Here's the drawing with two shaded views (mm, measured from the low corner). I have some questions. A direction names the side the tool comes from. Round coordinates to 2 decimals unless told otherwise and drop trailing zeros. Loops run counter-clockwise (first coordinate to the right, second up) from the corner with the lowest first, then second, coordinate; pieces in that order, holes last.
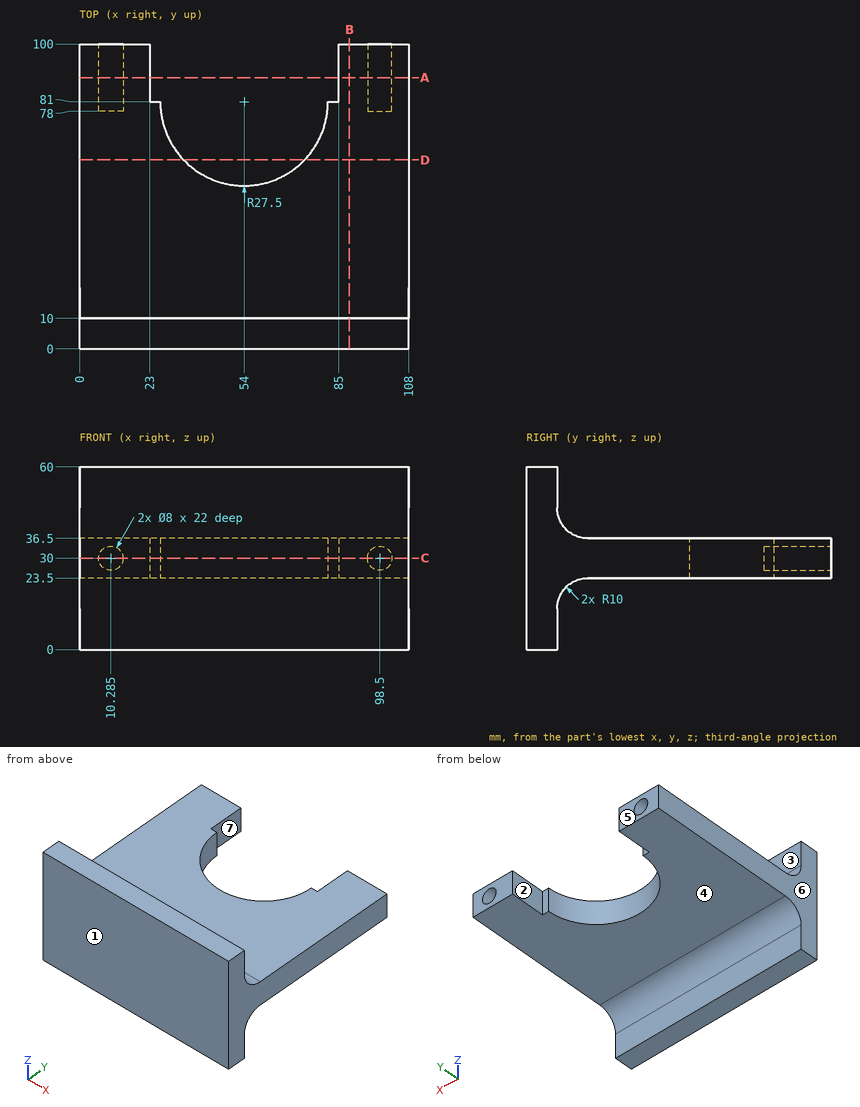
(1) If we section it at C-C, the plane z = 30: List the corners of the cut face in (x, y) for me (1 decimal).
Worked answers:
outline: (0, 0) - (108, 0) - (108, 100) - (102.5, 100) - (102.5, 78) - (94.5, 78) - (94.5, 100) - (85, 100) - (85, 81) - (81.5, 81) arc R27.5 cw to (26.5, 81) - (23, 81) - (23, 100) - (14.3, 100) - (14.3, 78) - (6.3, 78) - (6.3, 100) - (0, 100) - close
(2) If I drill on line 1 (Z direction, x = 98.5, y = 91.75); line 2 (Z direction, x = 101, y = 75.5); line 3 (Y direction, x = 68, z = 52.5), over which ranges is the centre line in solid material (lowest first)?
Worked answers:
line 1: z = 23.5 to 26, 34 to 36.5
line 2: z = 23.5 to 36.5
line 3: y = 0 to 10
(3) Will these pins go through, and if not, where does the flat tip stop? P1, Ø3, axis at x = 24, z = 27.5, coming from the +Y side; P2, Ø12, axis at x = 97, y = 18, coming from the +Z side; P3, Ø1.5, axis at x = 20, y = 37.5, coming from the -Z side; P4, Ø11, axis at x = 74.5, z = 55, coming from the +Y side.
Worked answers:
P1: stops at y = 100
P2: stops at z = 40.5
P3: stops at z = 23.5
P4: stops at y = 10
(4) If we mould it in two halves opening along X, with no side actions, what happens to the marked faces 5, 6 and 7? For each: released by +X, released by -X, zero draft, split by the parting line, or undercut.
Worked answers:
face 5: zero draft
face 6: released by -X
face 7: undercut
(5) If we section it at A-A, the plane y = 89: List the corners of the cut face in (x, z) for me (1 decimal).
Worked answers:
outline: (0, 23.5) - (23, 23.5) - (23, 36.5) - (0, 36.5) - close; (85, 23.5) - (108, 23.5) - (108, 36.5) - (85, 36.5) - close; hole circle Ø8 at (10.3, 30); hole circle Ø8 at (98.5, 30)
(6) If we section it at D-D, the plane y = 62: List the corners of the cut face in (x, z) for me.
Worked answers:
outline: (0, 23.5) - (34.12, 23.5) - (34.12, 36.5) - (0, 36.5) - close; (73.88, 23.5) - (108, 23.5) - (108, 36.5) - (73.88, 36.5) - close
(7) If we section it at B-B, the plane x = 88.5: List the corners of the cut face in (y, z) for me.
Worked answers:
outline: (0, 0) - (10, 0) - (10, 13.5) arc R10 cw to (20, 23.5) - (100, 23.5) - (100, 36.5) - (20, 36.5) arc R10 cw to (10, 46.5) - (10, 60) - (0, 60) - close
(8) For the marked faces 1, 2, 3 and 4, which set-ups out of +Z, -Z, +X, -X, +Y, -Y let a thin tool reach every point of the face, with its end or its side?
Worked answers:
face 1: +Z, -Z, +X, -X, -Y
face 2: +Z, -Z, +Y
face 3: +Z, +X, -X, +Y
face 4: -Z, +X, -X, +Y
